Design review of the part built by this model. Coordinates are the model's own, in mm. Face numbers are marked on the shaded views. A direction names the side the tool comes from. Round coordinates to 2 decimals unless told otherwise and drop trailing zeros. Order: outer loops, then holes, each group sorted by start corner. A loop starts at its lowest first (then second) coordinate and runs counter-clockwise, first axis right, second up.
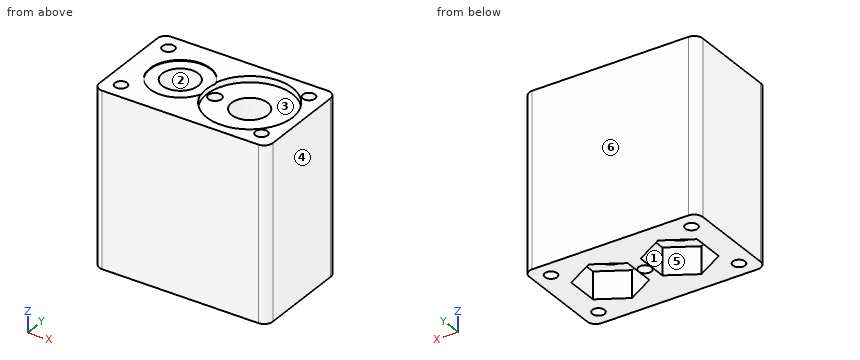
from build123d import *

# Parameters (mm, degrees)
SKETCH041_W     = 40
SKETCH041_H     = 24
PAD012_DEPTH    = 40
SKETCH042_R     = 4.15
HOLE017_DEPTH   = 50
SKETCH043_R     = 9.9
POCKET012_DEPTH = 1.4
POCKET021_DEPTH = 6.25
SKETCH066_R     = 1.4
HOLE026_DEPTH   = 50
SKETCH067_R     = 1.5
HOLE027_DEPTH   = 50
SKETCH068_R     = 7
POCKET022_DEPTH = 0.2
FILLET024_R     = 2


with BuildPart() as part:
    # Sketch041 → Pad012 (new body)
    with BuildSketch(Plane.XY):
        Rectangle(SKETCH041_W, SKETCH041_H)
    extrude(amount=PAD012_DEPTH)

    # Sketch042 (on Face6 of Pad012) → Hole017 (cut)
    with BuildSketch(Plane.XY.offset(40)):
        with Locations((8, 0)):
            Circle(SKETCH042_R)
    hole017 = extrude(amount=-HOLE017_DEPTH, mode=Mode.SUBTRACT)

    # Mirrored019: Hole017 across Sketch042 V_Axis
    add(hole017.mirror(Plane(origin=(0, 0, 40), x_dir=(0, 0, 1), z_dir=(1, 0, 0))), mode=Mode.SUBTRACT)

    # Sketch043 (on Face5 of Mirrored019) → Pocket012 (cut)
    with BuildSketch(Plane.XY.offset(40)):
        with Locations((8, 0)):
            Circle(SKETCH043_R)
    extrude(amount=-POCKET012_DEPTH, mode=Mode.SUBTRACT)

    # Sketch065 (on Face4 of Pocket012) → Pocket021 (cut)
    with BuildSketch(Plane(origin=(0, 0, 0), x_dir=(1, 0, 0), z_dir=(0, 0, -1))):
        Polygon((14.495191, 3.75), (8, 7.5), (1.504809, 3.75), (1.504809, -3.75), (8, -7.5), (14.495191, -3.75), align=None)
    pocket021 = extrude(amount=-POCKET021_DEPTH, mode=Mode.SUBTRACT)

    # Mirrored029: Pocket021 across Sketch065 V_Axis
    add(pocket021.mirror(Plane(origin=(0, 0, 0), x_dir=(0, 0, -1), z_dir=(1, 0, 0))), mode=Mode.SUBTRACT)

    # Sketch066 (on Face4 of Mirrored029) → Hole026 (cut)
    with BuildSketch(Plane(origin=(0, 0, 0), x_dir=(1, 0, 0), z_dir=(0, 0, -1))):
        with Locations((-16.2, 8.2)):
            Circle(SKETCH066_R)
        with Locations((-16.2, -8.2)):
            Circle(SKETCH066_R)
        with Locations((16.2, 8.2)):
            Circle(SKETCH066_R)
        with Locations((16.2, -8.2)):
            Circle(SKETCH066_R)
    extrude(amount=-HOLE026_DEPTH, mode=Mode.SUBTRACT)

    # Sketch067 (on Face4 of Hole026) → Hole027 (cut)
    with BuildSketch(Plane(origin=(0, 0, 0), x_dir=(1, 0, 0), z_dir=(0, 0, -1))):
        Circle(SKETCH067_R)
    extrude(amount=-HOLE027_DEPTH, mode=Mode.SUBTRACT)

    # Sketch068 (on Face5 of Hole027) → Pocket022 (cut)
    with BuildSketch(Plane.XY.offset(40)):
        with Locations((-8, 0)):
            Circle(SKETCH068_R)
    extrude(amount=-POCKET022_DEPTH, mode=Mode.SUBTRACT)

    # Fillet024
    fillet024_edges = [part.edges().sort_by_distance(p)[0] for p in [
        (20, 12, 20),
        (-20, 12, 20),
        (20, -12, 20),
        (-20, -12, 20),
    ]]
    fillet(fillet024_edges, radius=FILLET024_R)


solid = part.part
1) Clearance check with flat-ended pins moving along their axes: P1, Ø3, axis at x = 16.2, y = 8.2, coming from the +Z side; P2, Ø12, axis at x = 8, y = 0, coming from the +Z side; P3, Ø9.5, axis at x = -8, y = 0, coming from the -Z side; P4, Ø5, axis at x = 0, y = 0, coming from the +Z side. State where each tip first meets the part, or that it passes through.
Results:
P1: stops at z = 40
P2: stops at z = 38.6
P3: stops at z = 6.25
P4: stops at z = 39.8
2) Take a section at B-B on z = 12.5. Give the boundary of the cut face in (x, y), plus the area to 3 significant figures.
Results:
outline: (-20, -10) arc R2 ccw to (-18, -12) - (18, -12) arc R2 ccw to (20, -10) - (20, 10) arc R2 ccw to (18, 12) - (-18, 12) arc R2 ccw to (-20, 10) - close; hole circle Ø2.8 at (-16.2, -8.2); hole circle Ø2.8 at (-16.2, 8.2); hole circle Ø8.3 at (-8, 0); hole circle Ø3 at (0, 0); hole circle Ø8.3 at (8, 0); hole circle Ø2.8 at (16.2, -8.2); hole circle Ø2.8 at (16.2, 8.2)
area: 817 mm2
3) Take a section at D-D on x = 0. Give the boundary of the cut face in (y, z), plus the area to 3 significant figures.
Results:
outline: (-12, 0) - (-1.5, 0) - (-1.5, 38.6) - (-5.83, 38.6) - (-5.83, 40) - (-12, 40) - close; (1.5, 0) - (12, 0) - (12, 40) - (5.83, 40) - (5.83, 38.6) - (1.5, 38.6) - close
area: 828 mm2
4) For the marked faces 1, 2 and 3, list the 3-axis set-ups (+Z, -Z, +X, -X, +Y, -Y) from which the entire face can be reached by the end or side of a thin tool; tool diameter is ignored.
Results:
face 1: -Z
face 2: +Z, -Z
face 3: +Z
5) Take a section at A-A on x = -16.2. Give the boundary of the cut face in (y, z), plus the area to 3 significant figures.
Results:
outline: (-12, 0) - (-9.6, 0) - (-9.6, 40) - (-12, 40) - close; (-6.8, 0) - (6.8, 0) - (6.8, 40) - (-6.8, 40) - close; (9.6, 0) - (12, 0) - (12, 40) - (9.6, 40) - close
area: 736 mm2
6) The part is to be moulded in two halves that separate along X. For the marked faces 4, 5 and 6, say which applies: released by +X, released by -X, zero draft, split by the parting line, or undercut.
Results:
face 4: released by +X
face 5: undercut
face 6: zero draft
7) Take a section at C-C on y = 8.2. Give the boundary of the cut face in (x, z), plus the area to 3 significant figures.
Results:
outline: (-20, 0) - (-17.6, 0) - (-17.6, 40) - (-20, 40) - close; (-14.8, 0) - (14.8, 0) - (14.8, 40) - (13.55, 40) - (13.55, 38.6) - (2.45, 38.6) - (2.45, 40) - (-14.8, 40) - close; (17.6, 0) - (20, 0) - (20, 40) - (17.6, 40) - close
area: 1,360 mm2
8) To check wall thickness, follow line 1 along Y through (x, z) = (-16.2, 10); line 2 along X through (y, z) = (8.2, 15.5); line 3 along Y through (x, z) = (-8, 39.9). State the ranges of each line that lie inside material, in increasing order.
Results:
line 1: y = -12 to -9.6, -6.8 to 6.8, 9.6 to 12
line 2: x = -20 to -17.6, -14.8 to 14.8, 17.6 to 20
line 3: y = -12 to -7, 7 to 12
